from build123d import *

# Parameters (mm, degrees)
F1_DEPTH = 6.35
F2_W     = 2.54
F2_H     = 9.525
F3_DEPTH = 3.176
F4_W     = 2.54
F4_H     = 1.5875
F4_H_2   = 9.525
F5_DEPTH = 1.5748
F7_D     = 3.5814


with BuildPart() as f1:
    # F0 (on Front) → F1 (new body, symmetric)
    with BuildSketch(Plane.XZ):
        Polygon((0, 3.175), (0, 0), (31.115, 0), (31.115, 1.5875), (31.115, 3.175), align=None)
    extrude(amount=F1_DEPTH, both=True)

    # F2 (on face) → F3 (cut, through all)
    with BuildSketch(Plane.XY.offset(3.175)):
        with BuildLine():
            Line((28.575, -4.7625), (28.575, 4.7625))
            ThreePointArc((28.575, 4.7625), (25.2074039664, 3.3675960572), (23.8125, 3.35e-08))
            ThreePointArc((23.8125, 3.35e-08), (25.2074039428, -3.3675960336), (28.575, -4.7625))
        make_face()
        with Locations((29.845, 0)):
            Rectangle(F2_W, F2_H)
    extrude(amount=-F3_DEPTH, mode=Mode.SUBTRACT)

    # F4 (on face) → F5 (cut)
    with BuildSketch(Plane(origin=(0, 0, 0), x_dir=(1, 0, 0), z_dir=(0, 0, -1))):
        with Locations((29.845, 5.55625)):
            Rectangle(F4_W, F4_H)
        with Locations((29.845, 0)):
            Rectangle(F4_W, F4_H_2)
        with BuildLine():
            Line((28.575, 4.7625), (28.575, 6.35))
            ThreePointArc((28.575, 6.35), (24.0848719273, 4.4901280484), (22.225, -3.44e-08))
            ThreePointArc((22.225, -3.44e-08), (24.0848719516, -4.4901280727), (28.575, -6.35))
            Line((28.575, -6.35), (28.575, -4.7625))
            ThreePointArc((28.575, -4.7625), (23.8125, 0), (28.575, 4.7625))
        make_face()
        Polygon((31.115, -5.55625), (31.115, -4.7625), (28.575, -4.7625), (28.575, -6.35), (31.115, -6.35), align=None)
    extrude(amount=-F5_DEPTH, mode=Mode.SUBTRACT)

    # F7 (through all)
    with Locations(Plane.XY.offset(3.175)):
        with Locations((9.525, 0)):
            Hole(F7_D / 2)


solid = f1.part
Source: CAD feature listing. Evaluate the final solid. Frame: model axes, mm. A direction names the side the tool comes from. Round coordinates to 2 decimals unless told otherwise and drop trailing zeros. Order: outer loops, then holes, each group sorted by start corner. A loop starts at its lowest first (then second) coordinate and runs counter-clockwise, first axis right, second up. Notation, with made-up numbers: (83, -39.5) -> (129, -39.5) arc R9 cw to (129, -30.5) -> close; hole circle Ø5 at (17, -3.5). An arc over 180 degrees is marked (long way). Answer as CSV lines item,"result".
Item 1: Section C-C, the plane z = 0.7. Return loops of the section in (x, y) (3 decimals).
A:
outline,"(0, -6.35) -> (28.575, -6.35) arc R6.35 cw to (28.575, 6.35) -> (0, 6.35) -> close; hole circle Ø3.581 at (9.525, 0)"
Item 2: Reachability of faces 1 (the face through (30, -4.762, 2)), 2 (the face through (7.871, -0.686, 1.565)), 3 (the face through (23.7, -1, 1.575)) from +Z, -Z, +X, -X, +Y, -Y: full face, straight path, thin tool, end or side. Return the list, or none.
A:
face 1,"+Z, -Z, +X"
face 2,"+Z, -Z"
face 3,"-Z, +X"
Item 3: Section A-A, the plane x = 9.5. Return loops of the section in (y, z) (3 decimals).
A:
outline,"(-6.35, 0) -> (-1.791, 0) -> (-1.791, 3.175) -> (-6.35, 3.175) -> close; (1.791, 0) -> (6.35, 0) -> (6.35, 3.175) -> (1.791, 3.175) -> close"
Item 4: Pull-direction query (Y, two-part tool) for faces 4 (the face through (31.115, -6, 2)), 5 (the face through (30, 4.762, 2)), 6 (the face through (15, -6.35, 2)); classes: pulls with the +Y half, pulls with the -Y half, needs draft (parallel to the pull), parting line crosses it, or undercut.
A:
face 4,"needs draft"
face 5,"undercut"
face 6,"pulls with the -Y half"
Item 5: Line query: L1, parallel to Y at x = 10.5, z = 1.25; L2, parallel to X at y = -0.75, z = 2.4; L3, parallel to Y at x = 26, z = 2.6. Output: solid intervals per line, ascending.
A:
L1,"-6.35 to -1.5, 1.5 to 6.35"
L2,"0 to 7.9, 11.15 to 23.87"
L3,"-6.35 to -4.01, 4.01 to 6.35"
